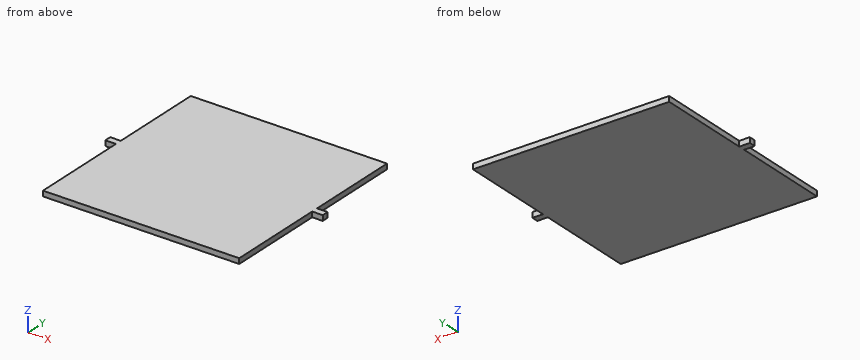
```python
from build123d import *

# Parameters (mm, degrees)
SKETCH_1_W      = 8
SKETCH_1_H      = 5
SKETCH_1_W_2    = 148
SKETCH_1_H_2    = 75
EXTRUDE_1_DEPTH = 4


with BuildPart() as part:
    # Эскиз1 → Бобышка-Вытянуть1 (new body)
    with BuildSketch(Plane.XY):
        Polygon((0, 80), (0, 75), (148, 75), (148, 80), (148, 152), (0, 152), align=None)
        with Locations((-4, 77.5)):
            Rectangle(SKETCH_1_W, SKETCH_1_H)
        with Locations((74, 37.5)):
            Rectangle(SKETCH_1_W_2, SKETCH_1_H_2)
        with Locations((152, 77.5)):
            Rectangle(SKETCH_1_W, SKETCH_1_H)
    extrude(amount=EXTRUDE_1_DEPTH)


solid = part.part
```
Can you work these out from the model? Positions are in its coordinate system, mm. Coordinates: 2 decimals unless noted, no trailing zeros. Loops run counter-clockwise (first coordinate to the right, second up) from the corner with the lowest first, then second, coordinate; pieces in that order, holes last. Notation, with made-up numbers: M -24,1 L -17,1 A19 ccw -17,36 Z; hole C 69.25,5.25 d7. An arc over 180 degrees is marked long. Put each result on its own line as item: value. Start each with the question number.
(1) Will these pins go through, and if not, where does the flat tip stop? pin 1 Ø1.2 at (x, z) = (-3, 2.5) entering from +Y; pin 2 Ø1.2 at (y, z) = (44, 2) entering from -X; pin 3 Ø2 at (y, z) = (119, 3) entering from +X.
(2) I need wall thicknesses on probe 1 along X at (y, z) = (145, 1.3). Which ranges of the line are inside material? Lowest first, please.
(3) Imagine slicing it at A-A on z = 2.55. List the corners of the cut face in (x, y) for me.
(4) Imagine slicing it at B-B on y = 51. List the corners of the cut face in (x, z) for me, and give its area (3 significant figures).
Worked answers:
1. pin 1: stops at y = 80
1. pin 2: stops at x = 0
1. pin 3: stops at x = 148
2. probe 1: x = 0 to 148
3. outline: M -8,75 L 0,75 L 0,0 L 148,0 L 148,75 L 156,75 L 156,80 L 148,80 L 148,152 L 0,152 L 0,80 L -8,80 Z
4. outline: M 0,0 L 148,0 L 148,4 L 0,4 Z
4. area: 592 mm2
